Geometry: final body of the model. Coordinates: model frame, mm. Face numbers are marked on the shaded views. A direction names the side the tool comes from. Give positions to 0.01 mm unless a question says otherwise; leave off trailing zeros. Loops run counter-clockwise (first coordinate to the right, second up) from the corner with the lowest first, then second, coordinate; pieces in that order, holes last. Notation, with made-up numbers: (7, 68.25) - (18, 68.25) arc R16 cw to (18, 73.25) - close; hole circle Ø8 at (63.5, 59). An arc over 180 degrees is marked (long way). Answer in a Markdown table with one row per item.
Autodesk Inventor part; units mm, degrees
ref_plane "Work Plane2" through (2.032, 0, 0) normal (0, 1, 0) x (1, 0, 0)
ref_plane "YZ Plane" through (0, 0, 0) normal (1, 0, 0) x (0, 1, 0)
ref_plane "XZ Plane" through (0, 0, 0) normal (0, 1, 0) x (-1, 0, 0)
sketch "Sketch1" plane through (0, 0, 0) normal (0, 0, 1) x (1, 0, 0)
  line L0 (2.2606, 0) -> (11.1125, 0)
  line L1 (11.1125, 0) -> (11.1125, 1.4224)
  line L2 (11.1125, 1.4224) -> (1.7018, 1.4224)
  line L3 (0.4892, 2.4765) -> (0, 2.4765)
  line L4 (-2.2225, 0) -> (13.335, 0)
  line L5 (0, -0.4953) -> (0, 2.9718)
  line L6 (0, 1.6256) -> (1.8999, 0.6783)
  line L7 (1.8999, 0.6783) -> (2.2606, 0)
  line L8 (1.7018, 1.4224) -> (0.4892, 2.4765)
  line L9 (0, 2.4765) -> (0, 1.6256)
  dimension "d2" = 2.8448
  dimension "d3" = 4.953
  dimension "d4" = 2.2606
  dimension "d5" = 3.2512
  dimension "d6" = 26.5
  dimension "d7" = 62
  dimension "d13" = 41
  dimension "d14" = 1.7018
  dimension "d15" = 11.1125
revolve "Body" add sketch "Sketch1" angle 360 about axis through (2.2606, 0, 0) along (1, 0, 0) contours L7 L6 L5 L3 L8 L2 L1 L0
sketch "Sketch2" plane through (0, 0, 0) normal (-1, 0, 0) x (0, 0, 1)
  line L0 (0, -3.4671) -> (0, 3.4671)
  line L1 (-3.4671, 0) -> (3.4671, 0)
  line L2 (0, 1.6256) -> (0, 0) construction
  line L3 (0, 0) -> (1.6256, 0) construction
  arc A0 (0.5419, 0) -> (0, 0.5419) centre (0, 0) ccw
  line L4 (0, 0) -> (0.7947, 0.7947) construction
  arc A1 (0.8128, 0) -> (0, 0.8128) centre (0, 0) ccw construction
  line L5 (0.2286, 1.6094) -> (0.2202, 0.7824)
  line L6 (1.6094, 0.2286) -> (0.7824, 0.2202)
  arc A2 (0.2202, 0.7824) -> (0.7824, 0.2202) centre (0.7767, 0.7767) ccw
  arc A3 (1.6256, 0) -> (1.6094, 0.2286) centre (0, 0) ccw
  arc A4 (0.2286, 1.6094) -> (0, 1.6256) centre (0, 0) ccw
  arc A5 (1.6094, 0.2286) -> (0.2286, 1.6094) centre (0, 0) ccw
  line L7 (0.2286, -1.6094) -> (0.2202, -0.7824)
  line L8 (1.6094, -0.2286) -> (0.7824, -0.2202)
  arc A6 (0.7824, -0.2202) -> (0.2202, -0.7824) centre (0.7767, -0.7767) ccw
  arc A7 (1.6094, -0.2286) -> (1.6256, 0) centre (0, 0) ccw
  arc A8 (0, -1.6256) -> (0.2286, -1.6094) centre (0, 0) ccw
  arc A9 (0.2286, -1.6094) -> (1.6094, -0.2286) centre (0, 0) ccw
  line L9 (-0.2286, 1.6094) -> (-0.2202, 0.7824)
  line L10 (-1.6094, 0.2286) -> (-0.7824, 0.2202)
  arc A10 (-0.7824, 0.2202) -> (-0.2202, 0.7824) centre (-0.7767, 0.7767) ccw
  arc A11 (-1.6094, 0.2286) -> (-1.6256, 0) centre (0, 0) ccw
  arc A12 (0, 1.6256) -> (-0.2286, 1.6094) centre (0, 0) ccw
  arc A13 (-0.2286, 1.6094) -> (-1.6094, 0.2286) centre (0, 0) ccw
  arc A14 (-1.6094, -0.2286) -> (-0.2286, -1.6094) centre (0, 0) ccw
  arc A15 (-0.2286, -1.6094) -> (0, -1.6256) centre (0, 0) ccw
  arc A16 (-1.6256, 0) -> (-1.6094, -0.2286) centre (0, 0) ccw
  line L11 (-1.6094, -0.2286) -> (-0.7824, -0.2202)
  arc A17 (-0.2202, -0.7824) -> (-0.7824, -0.2202) centre (-0.7767, -0.7767) ccw
  line L12 (-0.2286, -1.6094) -> (-0.2202, -0.7824)
  dimension "d18" = 45
  dimension "d19" = 1.0837
  dimension "d20" = 1.6256
  dimension "d21" = 3.2512
  dimension "d22" = 0.2286
extrude "Slot" add sketch "Sketch2" against normal up to next contours A2 L5 A5 L6 | L9 A10 L10 A13 | L7 A6 L8 A9 | A14 L11 A17 L12
fillet "Fillet1" radius 0.0914 4 edges at (0, 1.6256, 0) (0, 0, 1.6256) (0, -1.6256, 0) (0, 0, -1.6256)
thread "Thread"
chamfer "Chamfer1" distance 0.4763 distance2 0.4763 1 edges at (11.1125, -1.4224, 0) measured on face at (11.1125, 0.2736, 0.8712)
ref_plane "Work Plane2" through (2.032, 0, 0) normal (0, 1, 0) x (1, 0, 0)
equation "\"d2\" = GD"
equation "\"d3\" = KOD"
equation "\"d4\" = INTI"
equation "\"d5\" = SDM"
equation "\"d13\" = 0.5 * SEWI"
equation "\"d14\" = KOH"
equation "\"d15\" = NLG"
equation "\"d19\" = 0.333333 * SDM"
equation "\"d20\" = 0.5 * SDM"
equation "\"d21\" = SDM"
equation "\"d22\" = 0.5 * SBR"
equation "\"d45\" = INTI"
equation "\"d25\" = 0.2 * SBR"
equation "\"d9\" = GEL"
equation "\"d11\" = -0.5 * SPD + 0.5 * GD"
equation "\"d12\" = GUL"
equation "\"GD\" = NND"
equation "\"NLG\" = 11.1125"
equation "\"GEL\" = 7.8232"
equation "\"KOD\" = 4.953"
equation "\"KOH\" = 1.7018"
equation "\"SDM\" = 3.2512"
equation "\"INTI\" = 2.2606"
equation "\"SBR\" = 0.4572"
equation "\"GUL\" = 0.75 * GAL"
equation "\"SPD\" = 1.8923"
equation "\"SEWI\" = 82deg"
equation "\"d0\" = NLG"
equation "\"d1\" = KOH"
equation "\"d17\" = SDM"
equation "\"TOA\" = 30deg"
equation "\"THREADDIA\" = 2.8448"
equation "\"BDM\" = NND"
equation "\"NND\" = 2.8448"
equation "\"GAL\" = 0.635"
equation "\"GD1\" = SPD"
properties part number "ANSI B18.6.3 - 4-40 x 7/16, CRFCHMSTII(5)" material "Steel, Mild"
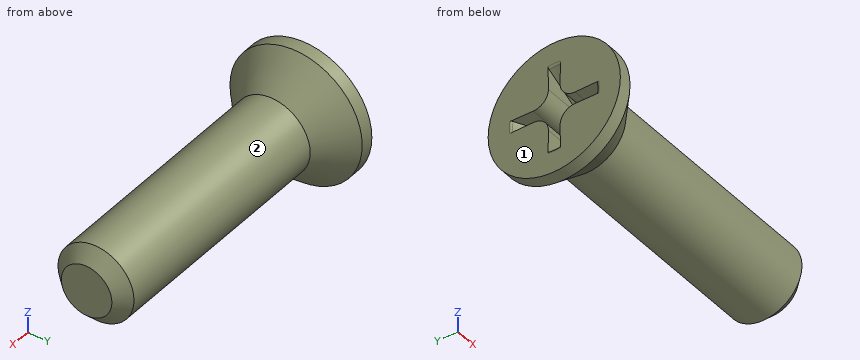
Q1. First-contact query: pin 1 (1.5 mm diameter, centred on x = 1.5, y = 0, fed in from -Z). Flat tip, straight axial feed; report the tip coordinate or a pass-through.
Check values:
| item | result |
|---|---|
| pin 1 | z = -2.25 |
Q2. Cut plane A-A (x = 3.25). Output: boundary loops of the cut face in (y, z).
Check values:
| item | result |
|---|---|
| outline | circle Ø2.84 at (0, 0) |
Q3. Reachability of the marked faces 1 and 2 from +Z, -Z, +X, -X, +Y, -Y: full face, straight path, thin tool, end or side. Return the list, or none.
Check values:
| item | result |
|---|---|
| face 1 | +Z, -Z, -X, +Y, -Y |
| face 2 | +X |
Q4. Material intervals for line 1 along Y through (x, z) = (9.75, 1.25); line 2 along X through (y, z) = (-1.1, -1.25); line 3 along X through (y, z) = (1.5, -1.9), sorted ascending.
Check values:
| item | result |
|---|---|
| line 1 | -0.68 to 0.68 |
| line 2 | 0 to 1.42 |
| line 3 | 0 to 0.55 |
